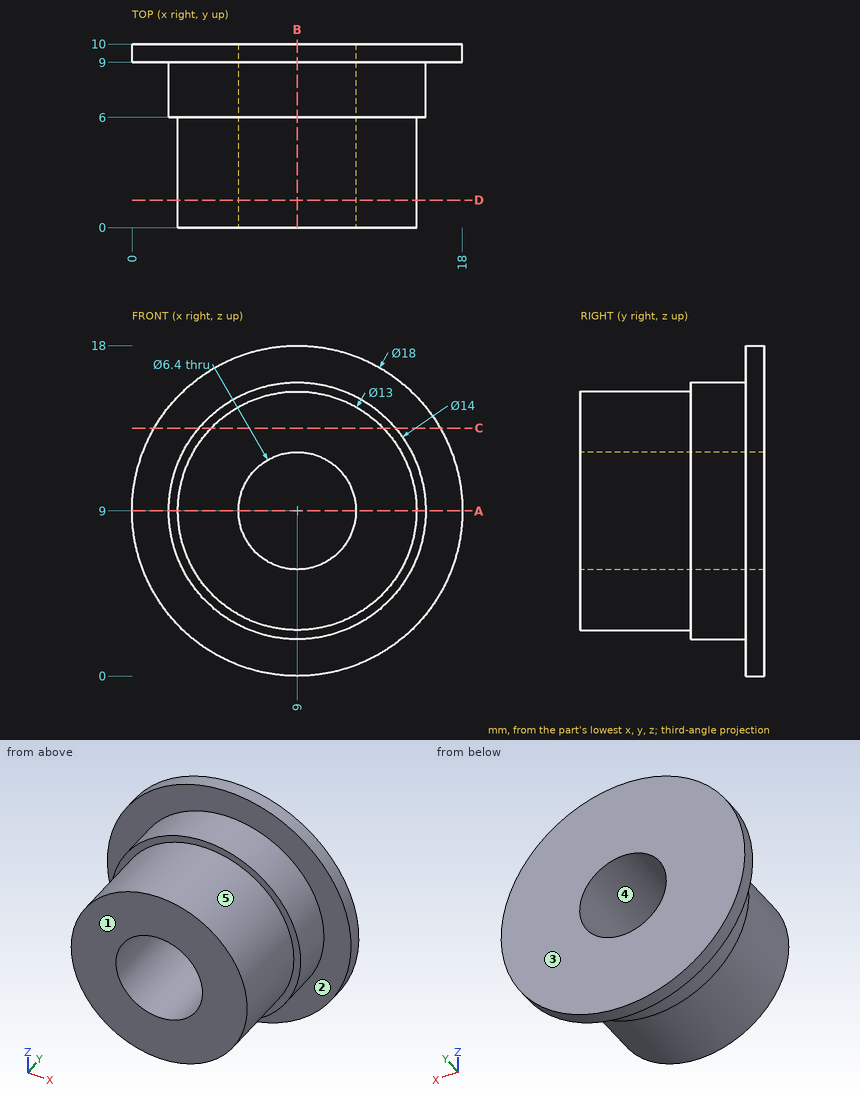
For this review, use the dimensioned drawing (mm, ordinates from the lowest corner) and the shaded views. A direction names the side the tool comes from. Round coordinates to 2 decimals unless told otherwise and drop trailing zeros. Order: outer loops, then holes, each group sorted by start corner. A loop starts at its lowest first (then second) coordinate and runs counter-clockwise, first axis right, second up. Notation, with made-up numbers: (5, 81) -> (20, 81) arc R18 ccw to (20, 89) -> close; hole circle Ø11 at (7, 68.5). An arc over 180 degrees is marked (long way). One line per item, written item: value. Start each with the question number.
Q1. Mouldability with a two-part tool opening along X and no side actions: class the marked faces 3, 4 and 5 as released by +X, released by -X, zero draft, split by the parting line, or undercut.
Q2. Machinability: for the marked faces 1 and 2, which of the approach directions +Z, -Z, +X, -X, +Y, -Y give a long, thin tool a straight path to every point of the face, cutting with its end or side? Answer none if there is none.
Q3. Take a section at D-D (y = 1.5). Write out the cut boundary in (x, z).
Q4. Take a section at C-C (z = 13.5). Write out the cut boundary in (x, y), and give its area (3 significant figures).
Q5. Take a section at A-A (z = 9). Write out the cut boundary in (x, y).
Q6. Wall thickness on line 1 (Z direction, x = 9, y = 6.75); line 2 (X direction, y = 4.5, z = 9): over which ranges is each line inside the solid? List them lowest first.
Q7. Take a section at B-B (x = 9). Write out the cut boundary in (y, z), and give its area (3 significant figures).
Q8. Clearance check with flat-ended pins moving along their axes: pin 1 Ø3 at (y, z) = (5, 8) entering from +X; pin 2 Ø6 at (y, z) = (5.5, 15.5) entering from -X; pin 3 Ø2 at (x, y) = (15.5, 2.5) entering from +Z. State where each tip first meets the part, or that it passes through.
Reported:
1. face 3: zero draft
1. face 4: undercut
1. face 5: split by the parting line
2. face 1: +Z, -Z, +X, -X, -Y
2. face 2: -Y
3. outline: circle Ø13 at (9, 9); hole circle Ø6.4 at (9, 9)
4. outline: (1.21, 9) -> (3.64, 9) -> (3.64, 6) -> (4.31, 6) -> (4.31, 0) -> (13.69, 0) -> (13.69, 6) -> (14.36, 6) -> (14.36, 9) -> (16.79, 9) -> (16.79, 10) -> (1.21, 10) -> close
4. area: 104 mm2
5. outline: (0, 9) -> (2, 9) -> (2, 6) -> (2.5, 6) -> (2.5, 0) -> (5.8, 0) -> (5.8, 10) -> (0, 10) -> close; (12.2, 0) -> (15.5, 0) -> (15.5, 6) -> (16, 6) -> (16, 9) -> (18, 9) -> (18, 10) -> (12.2, 10) -> close
6. line 1: z = 2 to 5.8, 12.2 to 16
6. line 2: x = 2.5 to 5.8, 12.2 to 15.5
7. outline: (0, 2.5) -> (6, 2.5) -> (6, 2) -> (9, 2) -> (9, 0) -> (10, 0) -> (10, 5.8) -> (0, 5.8) -> close; (0, 12.2) -> (10, 12.2) -> (10, 18) -> (9, 18) -> (9, 16) -> (6, 16) -> (6, 15.5) -> (0, 15.5) -> close
7. area: 74.0 mm2
8. pin 1: stops at x = 16
8. pin 2: stops at x = 2.96
8. pin 3: stops at z = 12.46
